The model under review builds one solid part; all positions refer to its coordinate system, in mm. Round coordinates to 2 decimals unless told otherwise and drop trailing zeros. Order: outer loops, then holes, each group sorted by start corner. A loop starts at its lowest first (then second) coordinate and runs counter-clockwise, first axis right, second up.
1) Consider section D-D (y = -52.5). Give the boundary of the cut face in (x, z), then the cut area to 3 significant figures.
2) Consider section C-C (z = -75). Give the boundary of the cut face in (x, y).
3) Consider section A-A (y = 88.5). Give the boundary of the cut face in (x, z).
4) Consider section B-B (x = 3.55). Give the number of separate pieces and of enclosed holes in the cut face, then the cut area to 3 significant figures.
5) To check wall thickness, follow L1, parallel to Z at x = 3.95, y = -46; L2, parallel to Y at x = 1.95, z = -114.3; L3, parallel to Y at x = 1, z = -218.5 (3 decimals). State the ranges of each line that lie inside material, in increasing order.
6) Clearance check with a flat-ended pin moving along its axis: P1, Ø5, axis at y = -146.81, z = -203.97, coming from the -X side. State where the tip first meets the part, or that it passes through.
from build123d import *

# Parameters (mm, degrees)
SKETCH1_W                 = 492.125
SKETCH1_H                 = 304.8
BOSS_EXTRUDE1_DEPTH       = 4.7625
CUT_EXTRUDE1_REACH        = 6.763
BOSS_EXTRUDE2_REACH       = 494.125
SKETCH3_W                 = 4.7625
SKETCH3_H                 = 304.8
F_8_CLEARANCE_HOLE1_D     = 4.3053
F_8_CLEARANCE_HOLE1_DEPTH = 74.422
F_8_CLEARANCE_HOLE1_TIP   = 1.293442612
SKETCH9_W                 = 381
SKETCH9_H                 = 215.9
CUT_EXTRUDE2_DEPTH        = 5.7625
F_8_CLEARANCE_HOLE2_D     = 4.4958
F_8_CLEARANCE_HOLE2_DEPTH = 74.422
F_8_CLEARANCE_HOLE2_TIP   = 1.350674586
F_6_CLEARANCE_HOLE1_D     = 3.7973
F_6_CLEARANCE_HOLE1_DEPTH = 74.422
F_6_CLEARANCE_HOLE1_TIP   = 1.140824014
SKETCH14_W                = 22.86
SKETCH14_H                = 46.99
CUT_EXTRUDE3_DEPTH        = 46.736


with BuildPart() as part:
    # Sketch1 → Boss-Extrude1 (new body)
    with BuildSketch(Plane(origin=(0, 0, 0), x_dir=(0, 0, -1), z_dir=(1, 0, 0))):
        Rectangle(SKETCH1_W, SKETCH1_H)
    extrude(amount=BOSS_EXTRUDE1_DEPTH)

    # Sketch2 → Cut-Extrude1 (cut, up to next)
    with BuildSketch(Plane(origin=(4.7625, 0, 0), x_dir=(0, 0, -1), z_dir=(1, 0, 0)), mode=Mode.PRIVATE) as cut_extrude1_sk1:
        Polygon((-24.852813742, -60), (24.852813742, -60), (42.426406871, -42.426406871), (60, -24.852813742), (60, 24.852813742), (24.852813742, 60), (-24.852813742, 60), (-60, 24.852813742), (-60, -24.852813742), align=None)
    cut_extrude1_tool1 = extrude(cut_extrude1_sk1.sketch, amount=-CUT_EXTRUDE1_REACH, mode=Mode.PRIVATE) & part.part
    add(cut_extrude1_tool1.solids().sort_by_distance((4.7625, 0, 0))[0], mode=Mode.SUBTRACT)

    # Sketch3 → Boss-Extrude2 (add, up to next)
    with BuildSketch(Plane.XY.offset(246.0625), mode=Mode.PRIVATE) as boss_extrude2_sk1:
        with Locations((2.38125, 0)):
            Rectangle(SKETCH3_W, SKETCH3_H)
    boss_extrude2_tool1 = extrude(boss_extrude2_sk1.sketch, amount=-BOSS_EXTRUDE2_REACH, mode=Mode.PRIVATE) - part.part
    add(boss_extrude2_tool1.solids().sort_by_distance((2.38125, 0, 246.0625))[0])

    # #8 Clearance Hole1
    with Locations(Plane(origin=(4.7625, 0, 0), x_dir=(0, 0, -1), z_dir=(1, 0, 0))):
        with Locations((-231.93375, -113.284), (-231.93375, -62.484), (231.93375, -62.484), (231.93375, -113.284)):
            Hole(F_8_CLEARANCE_HOLE1_D / 2, depth=F_8_CLEARANCE_HOLE1_DEPTH)
            with Locations((0, 0, -(F_8_CLEARANCE_HOLE1_DEPTH + F_8_CLEARANCE_HOLE1_TIP / 2))):  # 118° drill point
                Cone(0, F_8_CLEARANCE_HOLE1_D / 2, F_8_CLEARANCE_HOLE1_TIP, mode=Mode.SUBTRACT)

    # Sketch9 → Cut-Extrude2 (cut, through all)
    with BuildSketch(Plane(origin=(4.7625, 0, 0), x_dir=(0, 0, -1), z_dir=(1, 0, 0))):
        with Locations((0, -44.45)):
            Rectangle(SKETCH9_W, SKETCH9_H)
    extrude(amount=-CUT_EXTRUDE2_DEPTH, mode=Mode.SUBTRACT)

    # #8 Clearance Hole2
    with Locations(Plane(origin=(4.7625, 0, 0), x_dir=(0, 0, -1), z_dir=(1, 0, 0))):
        with Locations((-114.3, 73.81875), (-84.1375, 73.81875), (84.1375, 73.81875), (114.3, 73.81875)):
            Hole(F_8_CLEARANCE_HOLE2_D / 2, depth=F_8_CLEARANCE_HOLE2_DEPTH)
            with Locations((0, 0, -(F_8_CLEARANCE_HOLE2_DEPTH + F_8_CLEARANCE_HOLE2_TIP / 2))):  # 118° drill point
                Cone(0, F_8_CLEARANCE_HOLE2_D / 2, F_8_CLEARANCE_HOLE2_TIP, mode=Mode.SUBTRACT)

    # #6 Clearance Hole1
    with Locations(Plane(origin=(4.7625, 0, 0), x_dir=(0, 0, -1), z_dir=(1, 0, 0))):
        with Locations((-203.97089, -146.812), (203.97089, -146.812)):
            Hole(F_6_CLEARANCE_HOLE1_D / 2, depth=F_6_CLEARANCE_HOLE1_DEPTH)
            with Locations((0, 0, -(F_6_CLEARANCE_HOLE1_DEPTH + F_6_CLEARANCE_HOLE1_TIP / 2))):  # 118° drill point
                Cone(0, F_6_CLEARANCE_HOLE1_D / 2, F_6_CLEARANCE_HOLE1_TIP, mode=Mode.SUBTRACT)

    # Sketch14 → Cut-Extrude3 (cut)
    with BuildSketch(Plane(origin=(4.7625, 0, 0), x_dir=(0, 0, -1), z_dir=(1, 0, 0))):
        with Locations((218.1225, 78.74)):
            Rectangle(SKETCH14_W, SKETCH14_H)
    extrude(amount=-CUT_EXTRUDE3_DEPTH, mode=Mode.SUBTRACT)


solid = part.part
Answer below:
1. outline: (0, -246.06) - (4.76, -246.06) - (4.76, -190.5) - (0, -190.5) - close; (0, 190.5) - (4.76, 190.5) - (4.76, 246.06) - (0, 246.06) - close
1. area: 529 mm2
2. outline: (0, 63.5) - (4.76, 63.5) - (4.76, 152.4) - (0, 152.4) - close
3. outline: (0, -246.06) - (4.76, -246.06) - (4.76, -229.55) - (0, -229.55) - close; (0, -206.69) - (4.76, -206.69) - (4.76, 246.06) - (0, 246.06) - close
4. separate pieces: 1
4. enclosed holes: 11
4. area: 66,500 mm2
5. L1: z = -246.06 to -190.5, 190.5 to 246.06
5. L2: y = 63.5 to 71.57, 76.07 to 152.4
5. L3: y = -152.4 to 55.245, 102.235 to 152.4
6. P1: stops at x = 0
